Autodesk Inventor part; units mm, degrees
ref_plane "YZ Plane" through (0, 0, 0) normal (1, 0, 0) x (0, 1, 0)
ref_plane "XZ Plane" through (0, 0, 0) normal (0, 1, 0) x (-1, 0, 0)
ref_plane "XY Plane" through (0, 0, 0) normal (0, 0, 1) x (1, 0, 0)
ref_plane "Work Plane1" through (0, 0, 0) normal (0, 0, 1) x (1, 0, 0)
sketch "Sketch1" plane through (0, 0, 0) normal (0, 0, 1) x (1, 0, 0)
  line L0 (41.7899, 406.4) -> (106.8774, 406.4)
  line L1 (14.8024, 385.8381) -> (41.7899, 406.4)
  line L2 (106.8774, 403.225) -> (42.8616, 403.225)
  line L3 (42.8616, 403.225) -> (16.7266, 383.3126)
  line L4 (106.8774, 406.4) -> (106.8774, 403.225)
  line L5 (11.6274, 361.95) -> (11.6274, 80.1687)
  line L6 (16.7266, 383.3126) -> (11.6274, 379.4275)
  line L7 (14.8024, 385.8381) -> (8.4524, 381)
  line L8 (11.6274, 361.95) -> (11.6274, 379.4275)
  line L9 (11.6274, 361.95) -> (11.6274, 80.1687)
  line L10 (8.4524, 361.95) -> (8.4524, 80.1687)
  line L11 (11.6274, 361.95) -> (8.4524, 361.95)
  line L12 (8.4524, 361.95) -> (8.4524, 381)
  point P0 (0, 0)
  dimension "d0" = 3.175
extrude "Extrusion1" add sketch "Sketch1" along normal blind 387.35
properties part number "Drive BaseFront"
Can you work these out from the model? Positions are in its coordinate system, mm. A direction names the side the tool comes from. Give positions to 0.01 mm unless a question says otherwise; leave off trailing zeros. Order: outer loops, then holes, each group sorted by start corner. A loop starts at its lowest first (then second) coordinate and runs counter-clockwise, first axis right, second up. Notation, with made-up numbers: (89.5, 82) - (117.5, 82) arc R24 ccw to (117.5, 96) - close; hole circle Ø9 at (37, -20). An arc over 180 degrees is marked (long way). Use a Markdown table: item, result. Add a question column.
Q1. Please list where these lines run through material, in increasing order: line 1 along Y through (x, z) = (85, 290.5) (3 decimals); line 2 along X through (y, z) = (373, 163); line 3 along X through (y, z) = (393, 195).
Q2. If we section it at B-B on x = 59.5: Write out the boundary of the cut face in (y, z) (3 decimals), plus the area to 3 significant figures.
Q3. On a 3-axis mill with a long thin cutter (end or side, diameter ignored), from which of +Z, -Z, +X, -X, +Y, -Y can I reach the whole of each face in a straight line? I mean faces 1 (the flat face through (8.452, 371, 191)), 2 (the flat face through (75, 403.225, 191)). Say none if no direction works.
Q4. I'm going to push flat-ended pins straight in: pin 1 (8.5 mm diameter, centred on y = 374, z = 123, fed in from +X); pin 2 (6 mm diameter, centred on y = 390, z = 325, fed in from -X); pin 3 (2 mm diameter, centred on x = 55.5, z = 308.5, fed in from -Y) (3 decimals). Where does each tip first touch, or does it pass through?
Q5. If we section it at C-C on y = 369: Write out the boundary of the cut face in (x, z), plus the area to 3 significant figures.
Answers follow:
| question | item | result |
|---|---|---|
| 1 | line 1 | y = 403.225 to 406.4 |
| 1 | line 2 | x = 8.45 to 11.63 |
| 1 | line 3 | x = 24.2 to 29.44 |
| 2 | outline | (403.225, 0) - (406.4, 0) - (406.4, 387.35) - (403.225, 387.35) - close |
| 2 | area | 1,230 mm^2 |
| 3 | face 1 | +Z, -Z, -X, +Y, -Y |
| 3 | face 2 | +Z, -Z, +X, -Y |
| 4 | pin 1 | stops at x = 11.63 |
| 4 | pin 2 | stops at x = 16.33 |
| 4 | pin 3 | stops at y = 403.225 |
| 5 | outline | (8.45, 0) - (11.63, 0) - (11.63, 387.35) - (8.45, 387.35) - close |
| 5 | area | 1,230 mm^2 |
